```python
from build123d import *

# Parameters (mm, degrees)
F0_W     = 15
F0_H     = 60
F1_DEPTH = 50
F2_DEPTH = 20
F4_DEPTH = 15


with BuildPart() as f1:
    # F0 (on Front) → F1 (new body)
    with BuildSketch(Plane.XZ):
        with Locations((7.5, 30)):
            Rectangle(F0_W, F0_H)
    extrude(amount=F1_DEPTH)



with BuildPart() as f1b:
    # F0 (on Front) → F1, piece 2 (new body)
    with BuildSketch(Plane.XZ):
        Polygon((90, 31.4285714286), (90, 0), (110, 0), (110, 20), align=None)
    extrude(amount=F1_DEPTH)


with BuildPart() as f1_1:
    add(f1.part)

    add(f1b.part)  # F2 merges F1b
    # F0 (on Front) → F2 (join)
    with BuildSketch(Plane.XZ):
        Polygon((15, 60), (15, 0), (90, 0), (90, 31.4285714286), (40, 60), align=None)
    extrude(amount=F2_DEPTH)

    # F3 (on face) → F4 (cut)
    with BuildSketch(Plane.YZ.offset(15)):
        Polygon((-50, 60), (-50, 50), (-30, 60), align=None)
    extrude(amount=-F4_DEPTH, mode=Mode.SUBTRACT)


solid = f1_1.part
```
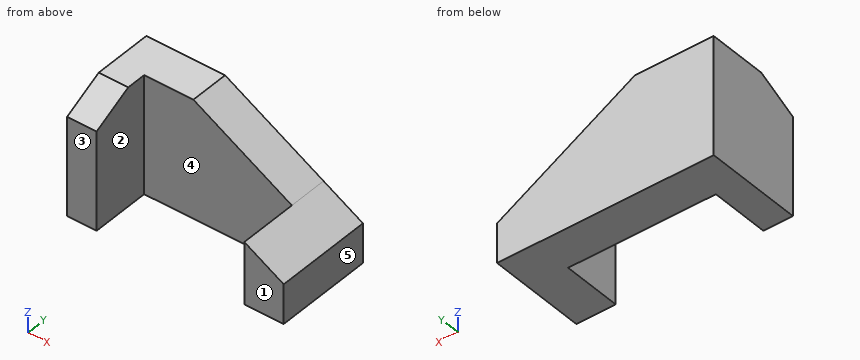
Geometry check sheet. Reference: the model listing, model coordinates, mm. Face numbers are marked on the shaded views. A direction names the side the tool comes from. Coordinates: 2 decimals unless noted, no trailing zeros. Loops run counter-clockwise (first coordinate to the right, second up) from the corner with the lowest first, then second, coordinate; pieces in that order, holes last. Notation, with made-up numbers: (36.25, 61) - (49.25, 61) arc R26 cw to (49.25, 77) - close; hole circle Ø7 at (-31, -7). An arc over 180 degrees is marked (long way). One line per item, written item: value. Start each with the question number.
(1) Cross-section at A-A on y = -23.5. Enter the section's corners in (x, z), plus the area to 3 significant figures.
(2) Tool access check on the marked faces 1 and 2. Record the directions out of +Z, -Z, +X, -X, +Y, -Y that give a thin tool (end or side, any length) a straight path to the whole face; none if there is none.
(3) Cross-section at B-B on z = 15. Enter the section's corners in (x, y), plus the area to 3 significant figures.
(4) Material ranges on line 1 (X direction, y = -21, z = 13); line 2 (Y direction, x = 81.5, z = 19); line 3 (X direction, y = -32.5, z = 52), recorded low to high. Write a range as [from, to].
(5) Cross-section at C-C on y = -46. Enter the section's corners in (x, z), plus the area to 3 significant figures.
(6) Mould release check, pull along X, two halves, no side actions. Record for the marked faces 3, 4 and 5: released by +X, released by -X, zero draft, split by the parting line, or undercut.
(7) Cross-section at D-D on x = 28.5. Enter the section's corners in (y, z), plus the area to 3 significant figures.
(8) Depth check by flat-ended pin: P1, Ø8, axis at y = -40, z = 40.5, coming from the +X side; P2, Ø3, axis at x = 17.5, y = -31, coming from the -Z side; P3, Ø8, axis at x = 73.5, y = -14.5, coming from the +Z side; P4, Ø18, axis at x = 52, z = 37, coming from the -Y side. Enter the tip coordinate at first touch or a pass-through.
Results below:
1. outline: (0, 0) - (15, 0) - (15, 60) - (0, 60) - close; (90, 0) - (110, 0) - (110, 20) - (90, 31.43) - close
1. area: 1,410 mm2
2. face 1: +Z, -Z, +X, -X, -Y
2. face 2: +Z, -Z, -Y
3. outline: (0, -50) - (15, -50) - (15, -20) - (90, -20) - (90, -50) - (110, -50) - (110, 0) - (0, 0) - close
3. area: 3,250 mm2
4. line 1: x = [0, 15], [90, 110]
4. line 2: y = [-20, 0]
4. line 3: x = [0, 15]
5. outline: (0, 0) - (15, 0) - (15, 52) - (0, 52) - close; (90, 0) - (110, 0) - (110, 20) - (90, 31.43) - close
5. area: 1,290 mm2
6. face 3: zero draft
6. face 4: undercut
6. face 5: released by +X
7. outline: (-20, 0) - (0, 0) - (0, 60) - (-20, 60) - close
7. area: 1,200 mm2
8. P1: stops at x = 15
8. P2: passes through
8. P3: stops at z = 43.14
8. P4: stops at y = -20
